from build123d import *

# Parameters (mm, degrees)
SKETCH1_R           = 2.55
BOSS_EXTRUDE1_DEPTH = 5
SKETCH_4_R          = 5
CUT_EXTRUDE_1_DEPTH = 2


with BuildPart() as part:
    # Sketch1 → Boss-Extrude1 (new body)
    with BuildSketch(Plane(origin=(0, 0, 0), x_dir=(1, 0, 0), z_dir=(0, 1, 0))):
        with BuildLine():
            Line((29.75, -32.75), (-29.75, -32.75))
            ThreePointArc((-29.75, -32.75), (-31.871320344, -31.871320344), (-32.75, -29.75))
            Line((-32.75, -29.75), (-32.75, 29.75))
            ThreePointArc((-32.75, 29.75), (-31.871320344, 31.871320344), (-29.75, 32.75))
            Line((-29.75, 32.75), (29.75, 32.75))
            ThreePointArc((29.75, 32.75), (31.871320344, 31.871320344), (32.75, 29.75))
            Line((32.75, 29.75), (32.75, -29.75))
            ThreePointArc((32.75, -29.75), (31.871320344, -31.871320344), (29.75, -32.75))
        make_face()
        with Locations(Location((0, 0, 0), (0, 0, 270))):
            Circle(SKETCH1_R, mode=Mode.SUBTRACT)
        with Locations(Location((10, -10, 0), (0, 0, 270))):
            Circle(SKETCH1_R, mode=Mode.SUBTRACT)
        with Locations(Location((20, -10, 0), (0, 0, 270))):
            Circle(SKETCH1_R, mode=Mode.SUBTRACT)
        with Locations(Location((10, -20, 0), (0, 0, 270))):
            Circle(SKETCH1_R, mode=Mode.SUBTRACT)
        with Locations(Location((20, -20, 0), (0, 0, 270))):
            Circle(SKETCH1_R, mode=Mode.SUBTRACT)
        with Locations(Location((-10, -10, 0), (0, 0, 270))):
            Circle(SKETCH1_R, mode=Mode.SUBTRACT)
        with Locations(Location((-20, -10, 0), (0, 0, 270))):
            Circle(SKETCH1_R, mode=Mode.SUBTRACT)
        with Locations(Location((-10, -20, 0), (0, 0, 270))):
            Circle(SKETCH1_R, mode=Mode.SUBTRACT)
        with Locations(Location((-20, -20, 0), (0, 0, 270))):
            Circle(SKETCH1_R, mode=Mode.SUBTRACT)
        with Locations(Location((0, -10, 0), (0, 0, 270))):
            Circle(SKETCH1_R, mode=Mode.SUBTRACT)
        with Locations(Location((0, -20, 0), (0, 0, 270))):
            Circle(SKETCH1_R, mode=Mode.SUBTRACT)
        with Locations(Location((10, 0, 0), (0, 0, 270))):
            Circle(SKETCH1_R, mode=Mode.SUBTRACT)
        with Locations(Location((20, 0, 0), (0, 0, 270))):
            Circle(SKETCH1_R, mode=Mode.SUBTRACT)
        with Locations(Location((10, 10, 0), (0, 0, 270))):
            Circle(SKETCH1_R, mode=Mode.SUBTRACT)
        with Locations(Location((20, 10, 0), (0, 0, 270))):
            Circle(SKETCH1_R, mode=Mode.SUBTRACT)
        with Locations(Location((10, 20, 0), (0, 0, 270))):
            Circle(SKETCH1_R, mode=Mode.SUBTRACT)
        with Locations(Location((20, 20, 0), (0, 0, 270))):
            Circle(SKETCH1_R, mode=Mode.SUBTRACT)
        with Locations(Location((-10, 0, 0), (0, 0, 270))):
            Circle(SKETCH1_R, mode=Mode.SUBTRACT)
        with Locations(Location((-20, 0, 0), (0, 0, 270))):
            Circle(SKETCH1_R, mode=Mode.SUBTRACT)
        with Locations(Location((-10, 10, 0), (0, 0, 270))):
            Circle(SKETCH1_R, mode=Mode.SUBTRACT)
        with Locations(Location((-20, 10, 0), (0, 0, 270))):
            Circle(SKETCH1_R, mode=Mode.SUBTRACT)
        with Locations(Location((-10, 20, 0), (0, 0, 270))):
            Circle(SKETCH1_R, mode=Mode.SUBTRACT)
        with Locations(Location((-20, 20, 0), (0, 0, 270))):
            Circle(SKETCH1_R, mode=Mode.SUBTRACT)
        with Locations(Location((0, 10, 0), (0, 0, 270))):
            Circle(SKETCH1_R, mode=Mode.SUBTRACT)
        with Locations(Location((0, 20, 0), (0, 0, 270))):
            Circle(SKETCH1_R, mode=Mode.SUBTRACT)
        with BuildLine():
            Line((-29.25, 16.75), (-29.25, 23.25))
            ThreePointArc((-29.25, 23.25), (-27.75, 24.75), (-26.25, 23.25))
            Line((-26.25, 23.25), (-26.25, 16.75))
            ThreePointArc((-26.25, 16.75), (-27.75, 15.25), (-29.25, 16.75))
        make_face(mode=Mode.SUBTRACT)
        with BuildLine():
            Line((26.25, 16.75), (26.25, 23.25))
            ThreePointArc((26.25, 23.25), (27.75, 24.75), (29.25, 23.25))
            Line((29.25, 23.25), (29.25, 16.75))
            ThreePointArc((29.25, 16.75), (27.75, 15.25), (26.25, 16.75))
        make_face(mode=Mode.SUBTRACT)
        with BuildLine():
            Line((3.25, 26.25), (-3.25, 26.25))
            ThreePointArc((-3.25, 26.25), (-4.75, 27.75), (-3.25, 29.25))
            Line((-3.25, 29.25), (3.25, 29.25))
            ThreePointArc((3.25, 29.25), (4.75, 27.75), (3.25, 26.25))
        make_face(mode=Mode.SUBTRACT)
        with BuildLine():
            Line((-16.75, 26.25), (-23.25, 26.25))
            ThreePointArc((-23.25, 26.25), (-24.75, 27.75), (-23.25, 29.25))
            Line((-23.25, 29.25), (-16.75, 29.25))
            ThreePointArc((-16.75, 29.25), (-15.25, 27.75), (-16.75, 26.25))
        make_face(mode=Mode.SUBTRACT)
        with BuildLine():
            Line((16.75, 26.25), (23.25, 26.25))
            ThreePointArc((23.25, 26.25), (24.75, 27.75), (23.25, 29.25))
            Line((23.25, 29.25), (16.75, 29.25))
            ThreePointArc((16.75, 29.25), (15.25, 27.75), (16.75, 26.25))
        make_face(mode=Mode.SUBTRACT)
        with BuildLine():
            Line((26.25, -3.25), (26.25, 3.25))
            ThreePointArc((26.25, 3.25), (27.75, 4.75), (29.25, 3.25))
            Line((29.25, 3.25), (29.25, -3.25))
            ThreePointArc((29.25, -3.25), (27.75, -4.75), (26.25, -3.25))
        make_face(mode=Mode.SUBTRACT)
        with BuildLine():
            Line((-16.75, -26.25), (-23.25, -26.25))
            ThreePointArc((-23.25, -26.25), (-24.75, -27.75), (-23.25, -29.25))
            Line((-23.25, -29.25), (-16.75, -29.25))
            ThreePointArc((-16.75, -29.25), (-15.25, -27.75), (-16.75, -26.25))
        make_face(mode=Mode.SUBTRACT)
        with BuildLine():
            Line((3.25, -26.25), (-3.25, -26.25))
            ThreePointArc((-3.25, -26.25), (-4.75, -27.75), (-3.25, -29.25))
            Line((-3.25, -29.25), (3.25, -29.25))
            ThreePointArc((3.25, -29.25), (4.75, -27.75), (3.25, -26.25))
        make_face(mode=Mode.SUBTRACT)
        with BuildLine():
            Line((16.75, -26.25), (23.25, -26.25))
            ThreePointArc((23.25, -26.25), (24.75, -27.75), (23.25, -29.25))
            Line((23.25, -29.25), (16.75, -29.25))
            ThreePointArc((16.75, -29.25), (15.25, -27.75), (16.75, -26.25))
        make_face(mode=Mode.SUBTRACT)
        with BuildLine():
            Line((26.25, -23.25), (26.25, -16.75))
            ThreePointArc((26.25, -16.75), (27.75, -15.25), (29.25, -16.75))
            Line((29.25, -16.75), (29.25, -23.25))
            ThreePointArc((29.25, -23.25), (27.75, -24.75), (26.25, -23.25))
        make_face(mode=Mode.SUBTRACT)
        with BuildLine():
            Line((-29.25, -3.25), (-29.25, 3.25))
            ThreePointArc((-29.25, 3.25), (-27.75, 4.75), (-26.25, 3.25))
            Line((-26.25, 3.25), (-26.25, -3.25))
            ThreePointArc((-26.25, -3.25), (-27.75, -4.75), (-29.25, -3.25))
        make_face(mode=Mode.SUBTRACT)
        with BuildLine():
            Line((-29.25, -23.25), (-29.25, -16.75))
            ThreePointArc((-29.25, -16.75), (-27.75, -15.25), (-26.25, -16.75))
            Line((-26.25, -16.75), (-26.25, -23.25))
            ThreePointArc((-26.25, -23.25), (-27.75, -24.75), (-29.25, -23.25))
        make_face(mode=Mode.SUBTRACT)
    extrude(amount=BOSS_EXTRUDE1_DEPTH)

    # 草圖4 → 除料-伸長1 (cut)
    with BuildSketch(Plane(origin=(0, 5, 0), x_dir=(1, 0, 0), z_dir=(0, 1, 0))):
        with Locations(Location((-20, -20, 0), (0, 0, 270))):
            Circle(SKETCH_4_R)
        with Locations(Location((20, -20, 0), (0, 0, 270))):
            Circle(SKETCH_4_R)
        with Locations(Location((20, 20, 0), (0, 0, 270))):
            Circle(SKETCH_4_R)
        with Locations(Location((-20, 20, 0), (0, 0, 270))):
            Circle(SKETCH_4_R)
    extrude(amount=-CUT_EXTRUDE_1_DEPTH, mode=Mode.SUBTRACT)


solid = part.part
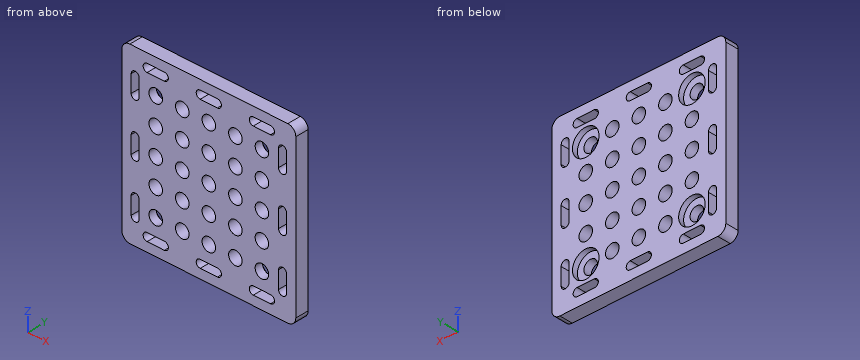
Can you work these out from the model? Positions are in its coordinate system, mm. Round coordinates to 2 decimals unless told otherwise and drop trailing zeros. Write each loop counter-clockwise with the first axis right and the second up, starting at its lowest first coordinate (ties: lowest second). Pieces come first, ordered by that corner, then holes. Notation, with made-up numbers: M 70.25,53 L 99.25,53 A33 ccw 99.25,84 Z; hole C 82.25,-34.75 d1. An arc over 180 degrees is marked long. Use a Markdown table: item, result.
Item 1: I want a section at A-A (x = 27.5). List the corners of the cut face in (y, z) for me.
Found:
| item | result |
|---|---|
| outline | M 0,-32.75 L 5,-32.75 L 5,-24.73 L 0,-24.73 Z; M 0,-15.27 L 5,-15.27 L 5,-4.73 L 0,-4.73 Z; M 0,4.73 L 5,4.73 L 5,15.27 L 0,15.27 Z; M 0,24.73 L 5,24.73 L 5,32.75 L 0,32.75 Z |
Item 2: I want a section at B-B (z = 1). State how many separate pieces and enclosed holes the cut face has, and give its area (3 significant figures).
Found:
| item | result |
|---|---|
| separate pieces | 8 |
| enclosed holes | 0 |
| area | 180 mm2 |
Item 3: If I drill on line 1 along X through (y, z) = (1.6, 10); line 2 along Z through (x, y) = (15.5, 4.1); line 3 along Z through (x, y) = (-23, 2.6), over which ranges is the centre line in solid material (lowest first)? Write a range as [from, to].
Found:
| item | result |
|---|---|
| line 1 | x = [-32.75, -22.55], [-17.45, -12.55], [-7.45, -2.55], [2.55, 7.45], [12.55, 17.45], [22.55, 32.75] |
| line 2 | z = [-32.75, -28.58], [-26.92, -22.18], [-17.82, 17.82], [22.18, 26.92], [28.58, 32.75] |
| line 3 | z = [-32.75, -29.25], [-26.25, 26.25], [29.25, 32.75] |
Item 4: For pin 1 Ø11 at (x, z) = (17.5, 18.5) entering from +Y, with a flat end and sliding along its axis, tell me the tip position at first contact or that it passes through.
Found:
| item | result |
|---|---|
| pin 1 | stops at y = 5 |
